```python
from build123d import *

# Parameters (mm, degrees)
BOSS_EXTRUDE1_DEPTH = 171.2
FILLET1_R           = 1
SKETCH2_R           = 1.8
CUT_EXTRUDE1_DEPTH  = 200
CUT_EXTRUDE2_DEPTH  = 2
LPATTERN1_COUNT     = 3
LPATTERN1_PITCH     = 116
CUT_EXTRUDE3_DEPTH  = 1


with BuildPart() as part:
    # Sketch1 → Boss-Extrude1 (new body)
    with BuildSketch(Plane.XY):
        Polygon((0, 0), (5.8, 0), (8.7, 3.9), (-2.9, 3.9), align=None)
    extrude(amount=BOSS_EXTRUDE1_DEPTH)

    # Fillet1
    fillet1_edges = [part.edges().sort_by_distance(p)[0] for p in [
        (-2.9, 3.9, 85.6),
        (8.7, 3.9, 85.6),
    ]]
    fillet(fillet1_edges, radius=FILLET1_R)

    # Sketch2 → Cut-Extrude1 (cut)
    with BuildSketch(Plane.XZ):
        with Locations(Location((2.9, 143.6, 0), (0, 0, 270))):
            Circle(SKETCH2_R)
    cut_extrude1 = extrude(amount=-CUT_EXTRUDE1_DEPTH, mode=Mode.SUBTRACT)

    # Sketch3 → Cut-Extrude2 (cut)
    with BuildSketch(Plane.XZ):
        Polygon((2.92874321, 146.948508199), (0.01447844, 145.29914645), (-0.014264771, 141.950638251), (2.87125679, 140.251491801), (5.78552156, 141.90085355), (5.814264771, 145.249361749), align=None)
    cut_extrude2 = extrude(amount=-CUT_EXTRUDE2_DEPTH, mode=Mode.SUBTRACT)

    # LPattern1: Cut-Extrude1, Cut-Extrude2 ×3
    with Locations(*[(0, 0, -i * LPATTERN1_PITCH) for i in range(1, LPATTERN1_COUNT)]):
        add(cut_extrude1, mode=Mode.SUBTRACT)
        add(cut_extrude2, mode=Mode.SUBTRACT)

    # Sketch4 → Cut-Extrude3 (cut)
    with BuildSketch(Plane(origin=(0, 3.9, 0), x_dir=(1, 0, 0), z_dir=(0, 1, 0))):
        Polygon((2.277474494, -98.3), (4.625651577, -98.3), (4.625651577, -85.6), (3.485907988, -85.6), (3.485907988, -96.997435897), (1.532061834, -96.997435897), align=None)
    extrude(amount=-CUT_EXTRUDE3_DEPTH, mode=Mode.SUBTRACT)


solid = part.part
```
Input: part model. Units: mm. Frame: model coordinates. A direction names the side the tool comes from. Round coordinates to 2 decimals unless told otherwise and drop trailing zeros. Loops run counter-clockwise (first coordinate to the right, second up) from the corner with the lowest first, then second, coordinate; pieces in that order, holes last.
1) Section query A-A on y = 1.4. Return the cut outline in (x, z), plus the area to 3 significant figures.
Ans:
outline: (-1.04, 0) - (6.84, 0) - (6.84, 171.2) - (-1.04, 171.2) - close; hole (-0.01, 25.95) - (2.87, 24.25) - (5.79, 25.9) - (5.81, 29.25) - (2.93, 30.95) - (0.01, 29.3) - close; hole (-0.01, 141.95) - (2.87, 140.25) - (5.79, 141.9) - (5.81, 145.25) - (2.93, 146.95) - (0.01, 145.3) - close
area: 1,290 mm2
2) Set-up query: faces 1 (the flat face through (1.56, 2, 26.16)), 2 (the cylindrical face through (2.98, 2.94, 145.4)). Return all of +Z, -Z, +X, -X, +Y, -Y with unobstructed straight access to the full face (end or side cutting, diameter ignored); none if empty.
Ans:
face 1: -Y
face 2: +Y, -Y
3) Pull-direction query (Z, two-part tool) for faces 3 (the flat face through (3, 2, 0)), 4 (the flat face through (3, 0, 157)), 5 (the cylindrical face through (4.418, 2.937, 26.632)), 6 (the flat face through (1.56, 2, 142.16)); classes: released by +Z, released by -Z, zero draft, split by the parting line, or undercut.
Ans:
face 3: released by -Z
face 4: zero draft
face 5: undercut
face 6: undercut
4) Material intervals for line 1 (Z direction, x = 5.75, y = 0.25); line 2 (X direction, y = 2.95, z = 27.6); line 3 (Z direction, x = 4.25, y = 0.2), sorted ascending.
Ans:
line 1: z = 0 to 25.88, 29.29 to 141.88, 145.29 to 171.2
line 2: x = -1.91 to 1.1, 4.7 to 7.71
line 3: z = 0 to 25.03, 30.17 to 141.03, 146.17 to 171.2
5) Section query B-B on z = 103. Return the cut outline in (x, y).
Ans:
outline: (-1.71, 2.3) - (0, 0) - (5.8, 0) - (7.51, 2.3) arc R1 ccw to (6.71, 3.9) - (-0.91, 3.9) arc R1 ccw to start
6) Pin query (flat end, axial travel): pin 1 (0.8 mm diameter, centred on y = 3.5, z = 88.5, fed in from +X); pin 2 (1.1 mm diameter, centred on x = 3.5, y = 3, fed in from -Z). Return the tip coordinate at first contact, or that it passes through.
Ans:
pin 1: stops at x = 7.69
pin 2: stops at z = 0
